Can you work these out from the model? Positions are in its coordinate system, mm. Round coordinates to 2 decimals unless told otherwise and drop trailing zeros. Loops run counter-clockwise (first coordinate to the right, second up) from the corner with the lowest first, then second, coordinate; pieces in that order, holes last. Notation, with made-up numbers: M -19.5,-26.75 L 21.5,-26.75 A4 ccw 21.5,-22.75 Z; hole C 11,42 d2. An arc over 180 degrees is marked long. Answer as CSV lines item,"result".
from build123d import *

# Parameters (mm, degrees)
SKETCH1_W               = 88.9
SKETCH1_H               = 203.2
BOSS_EXTRUDE1_DEPTH     = 6.35
SKETCH3_W               = 29.633333334
SKETCH3_H               = 6.35
CUT_EXTRUDE2_DEPTH      = 112.079633597
CAVITY2_START           = -101.6
CAVITY2_OUTLINE_W       = 6.35
CAVITY2_OUTLINE_H       = 6.35
CAVITY2_DEPTH           = 29.028571429
CAVITY2_START_2         = -43.542857143
CAVITY2_2_OUTLINE_W     = 6.35
CAVITY2_2_OUTLINE_H     = 6.35
CAVITY2_2_DEPTH         = 29.028571429
CAVITY2_START_3         = 14.514285714
CAVITY2_3_OUTLINE_W     = 6.35
CAVITY2_3_OUTLINE_H     = 6.35
CAVITY2_3_DEPTH         = 29.028571429
CUT_EXTRUDE3_DEPTH      = 112.079633597
SKETCH5_W               = 38.1
SKETCH5_H               = 163.83
BOSS_EXTRUDE2_DEPTH     = 6.35
CAVITY3_START           = 49.53
CAVITY3_OUTLINE_W       = 25.4
CAVITY3_OUTLINE_H       = 6.35
CAVITY3_DEPTH           = 6.35
CAVITY3_START_2         = -101.6
CAVITY3_2_OUTLINE_W     = 6.35
CAVITY3_2_OUTLINE_H     = 6.35
CAVITY3_2_DEPTH         = 29.028571429
CAVITY3_START_3         = -43.542857143
CAVITY3_3_OUTLINE_W     = 6.35
CAVITY3_3_OUTLINE_H     = 6.35
CAVITY3_3_DEPTH         = 29.028571429
CAVITY3_START_4         = 14.514285714
CAVITY3_4_OUTLINE_W     = 6.35
CAVITY3_4_OUTLINE_H     = 6.35
CAVITY3_4_DEPTH         = 29.028571429
SKETCH7_W               = 127
SKETCH7_H               = 6.35
CUT_EXTRUDE4_DEPTH      = 132.062523247
CUT_EXTRUDE5_DEPTH      = 132.062523247
CUT_EXTRUDE5_DEPTH_BACK = 132.062523247
SKETCH9_R               = 1.3716
CUT_EXTRUDE6_DEPTH      = 132.062523247
SKETCH10_R              = 2.286
CUT_EXTRUDE8_DEPTH      = 132.062523247


# Read off the part's stored shape, not the designer's step: Cavity2, Cavity3
with BuildPart() as part:
    # Sketch1 → Boss-Extrude1 (new body)
    with BuildSketch(Plane.XY):
        Rectangle(SKETCH1_W, SKETCH1_H)
    extrude(amount=BOSS_EXTRUDE1_DEPTH)

    # Sketch3 → Cut-Extrude2 (cut, through all)
    with BuildSketch(Plane(origin=(0, 0, 0), x_dir=(-1, 0, 0), z_dir=(0, 0, -1))):
        with Locations((0, -98.425)):
            Rectangle(SKETCH3_W, SKETCH3_H)
    extrude(amount=-CUT_EXTRUDE2_DEPTH, mode=Mode.SUBTRACT)

    # Cavity2 outline → Cavity2 (cut)
    with BuildSketch(Plane(origin=(0, 0, 0), x_dir=(1, 0, 0), z_dir=(0, 1, 0)).offset(CAVITY2_START)):
        with Locations((41.275, -3.175)):
            Rectangle(CAVITY2_OUTLINE_W, CAVITY2_OUTLINE_H)
    extrude(amount=CAVITY2_DEPTH, mode=Mode.SUBTRACT)

    # Cavity2 2 outline → Cavity2 2 (cut)
    with BuildSketch(Plane(origin=(0, 0, 0), x_dir=(1, 0, 0), z_dir=(0, 1, 0)).offset(CAVITY2_START_2)):
        with Locations((41.275, -3.175)):
            Rectangle(CAVITY2_2_OUTLINE_W, CAVITY2_2_OUTLINE_H)
    extrude(amount=CAVITY2_2_DEPTH, mode=Mode.SUBTRACT)

    # Cavity2 3 outline → Cavity2 3 (cut)
    with BuildSketch(Plane(origin=(0, 0, 0), x_dir=(1, 0, 0), z_dir=(0, 1, 0)).offset(CAVITY2_START_3)):
        with Locations((41.275, -3.175)):
            Rectangle(CAVITY2_3_OUTLINE_W, CAVITY2_3_OUTLINE_H)
    extrude(amount=CAVITY2_3_DEPTH, mode=Mode.SUBTRACT)

    # Sketch4 → Cut-Extrude3 (cut, through all)
    with BuildSketch(Plane(origin=(0, 0, 0), x_dir=(-1, 0, 0), z_dir=(0, 0, -1))):
        Polygon((0, 62.23), (44.45, 62.23), (44.45, 101.6), (-44.45, 101.6), (-44.45, 62.23), align=None)
    extrude(amount=-CUT_EXTRUDE3_DEPTH, mode=Mode.SUBTRACT)

    # Sketch5 → Boss-Extrude2 (add, through all)
    with BuildSketch(Plane(origin=(0, 0, 0), x_dir=(-1, 0, 0), z_dir=(0, 0, -1))):
        with Locations((63.5, -19.685)):
            Rectangle(SKETCH5_W, SKETCH5_H)
    extrude(amount=-BOSS_EXTRUDE2_DEPTH)

    # Cavity3 outline → Cavity3 (cut)
    with BuildSketch(Plane(origin=(0, 0, 0), x_dir=(1, 0, 0), z_dir=(0, 1, 0)).offset(CAVITY3_START)):
        with Locations((-69.85, -3.175)):
            Rectangle(CAVITY3_OUTLINE_W, CAVITY3_OUTLINE_H)
        with Locations((-19.05, -3.175)):
            Rectangle(CAVITY3_OUTLINE_W, CAVITY3_OUTLINE_H)
        with Locations((31.75, -3.175)):
            Rectangle(CAVITY3_OUTLINE_W, CAVITY3_OUTLINE_H)
    extrude(amount=CAVITY3_DEPTH, mode=Mode.SUBTRACT)

    # Cavity3 2 outline → Cavity3 2 (cut)
    with BuildSketch(Plane(origin=(0, 0, 0), x_dir=(1, 0, 0), z_dir=(0, 1, 0)).offset(CAVITY3_START_2)):
        with Locations((-79.375, -3.175)):
            Rectangle(CAVITY3_2_OUTLINE_W, CAVITY3_2_OUTLINE_H)
    extrude(amount=CAVITY3_2_DEPTH, mode=Mode.SUBTRACT)

    # Cavity3 3 outline → Cavity3 3 (cut)
    with BuildSketch(Plane(origin=(0, 0, 0), x_dir=(1, 0, 0), z_dir=(0, 1, 0)).offset(CAVITY3_START_3)):
        with Locations((-79.375, -3.175)):
            Rectangle(CAVITY3_3_OUTLINE_W, CAVITY3_3_OUTLINE_H)
    extrude(amount=CAVITY3_3_DEPTH, mode=Mode.SUBTRACT)

    # Cavity3 4 outline → Cavity3 4 (cut)
    with BuildSketch(Plane(origin=(0, 0, 0), x_dir=(1, 0, 0), z_dir=(0, 1, 0)).offset(CAVITY3_START_4)):
        with Locations((-79.375, -3.175)):
            Rectangle(CAVITY3_4_OUTLINE_W, CAVITY3_4_OUTLINE_H)
    extrude(amount=CAVITY3_4_DEPTH, mode=Mode.SUBTRACT)

    # Sketch7 → Cut-Extrude4 (cut, through all)
    with BuildSketch(Plane(origin=(0, 0, 0), x_dir=(-1, 0, 0), z_dir=(0, 0, -1))):
        with Locations((19.05, 59.055)):
            Rectangle(SKETCH7_W, SKETCH7_H)
    extrude(amount=-CUT_EXTRUDE4_DEPTH, mode=Mode.SUBTRACT)

    # Sketch8 → Cut-Extrude5 (cut, two sides: drawn at the far end of the back side and taken through both)
    with BuildSketch(Plane(origin=(0, 0, 0), x_dir=(-1, 0, 0), z_dir=(0, 0, -1)).offset(-CUT_EXTRUDE5_DEPTH_BACK)):
        Polygon((51.816, -480.745462689), (51.816, -101.6), (51.816, -95.25), (22.098, -95.25), (22.098, -101.6), (22.098, -480.745462689), (22.098, -1239.036388068), (51.816, -1239.036388068), align=None)
    extrude(amount=CUT_EXTRUDE5_DEPTH + CUT_EXTRUDE5_DEPTH_BACK, mode=Mode.SUBTRACT)

    # Sketch9 → Cut-Extrude6 (cut, through all)
    with BuildSketch(Plane.XY.offset(6.35)):
        with Locations((-55.88, -63.5)):
            Circle(SKETCH9_R)
        with Locations((17.78, -69.342)):
            Circle(SKETCH9_R)
        with Locations((-55.88, -10.16)):
            Circle(SKETCH9_R)
        with Locations((17.78, -3.302)):
            Circle(SKETCH9_R)
    extrude(amount=-CUT_EXTRUDE6_DEPTH, mode=Mode.SUBTRACT)

    # Sketch10 → Cut-Extrude8 (cut, through all)
    with BuildSketch(Plane(origin=(0, 0, 0), x_dir=(-1, 0, 0), z_dir=(0, 0, -1))):
        with Locations((61.309312367, -72.22311472)):
            Circle(SKETCH10_R)
        with Locations((63.059030347, 0.028511897)):
            Circle(SKETCH10_R)
        with Locations((-23.90939041, -72.710988475)):
            Circle(SKETCH10_R)
        with Locations((-25.303227794, -0.994316453)):
            Circle(SKETCH10_R)
    extrude(amount=-CUT_EXTRUDE8_DEPTH, mode=Mode.SUBTRACT)


solid = part.part
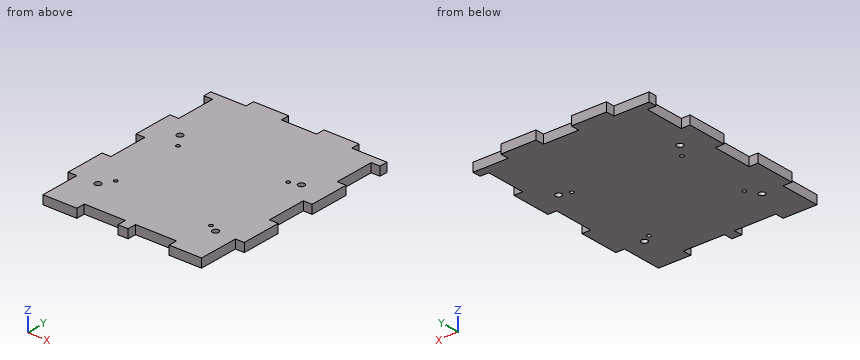
Item 1: If I drill on line 1 along Y through (x, z) = (17.78, 5); line 2 along X through (y, z) = (-74, 2.25); line 3 along Y through (x, z) = (38, 2), over which ranges is the centre line in solid material (lowest first)? Write a range as from..to.
Output:
line 1,"y = -101.6..-70.71, -67.97..-4.67, -1.93..55.88"
line 2,"x = -76.2..-62.75, -59.87..22.02, 25.8..38.1"
line 3,"y = -101.6..49.53"
Item 2: If we section it at A-A on y = 28.5: Write out the boundary of the cut face in (x, z), then the cut area to 3 significant figures.
Output:
outline,"M -76.2,0 L 38.1,0 L 38.1,6.35 L -76.2,6.35 Z"
area,"726 mm2"
Item 3: If we section it at B-B on z = 3: State how many separate pieces and enclosed holes the cut face has, then the cut area to 3 significant figures.
Output:
separate pieces,"1"
enclosed holes,"8"
area,"17,900 mm2"
Item 4: Will these pins go through, and if not, where does the flat tip stop? pin 1 (2 mm diameter, centred on y = 30, z = 5, fed in from -X); pin 2 (1.9 mm diameter, centred on y = 52, z = 2.5, fed in from -X); pin 3 (3 mm diameter, centred on y = -97.5, z = 2.5, fed in from +X).
Output:
pin 1,"stops at x = -76.2"
pin 2,"stops at x = -57.15"
pin 3,"stops at x = 38.1"
